Design review of the part built by this model. Coordinates are the model's own, in mm. A direction names the side the tool comes from. Round coordinates to 2 decimals unless told otherwise and drop trailing zeros. Order: outer loops, then holes, each group sorted by start corner. A loop starts at its lowest first (then second) coordinate and runs counter-clockwise, first axis right, second up. Notation, with made-up numbers: M 79,22 L 122,22 A12 ccw 122,26 Z; hole C 58,16.5 d4. An arc over 180 degrees is marked long. Use a Markdown table: item, result. Add a question column.
(1) Machinability: for faces 1 (the face through (26.877, 0.986, 63.376)), 2 (the face through (-36.96, 0.99, 55.82)), which of the approach directions +Z, -Z, +X, -X, +Y, -Y give a long, thin tool a straight path to every point of the face, cutting with its end or side? Answer none if there is none.
(2) Take a section at B-B (z = 11). Write out the cut boundary in (x, y) (3 decimals), then the cut area to 3 significant figures.
(3) Take a section at A-A (x = 47). Write out the cut boundary in (y, z), then the cut area to 3 significant figures.
(4) Take a section at D-D (y = 1.6). Count the separate pieces of the cut face and the enclosed holes in it, then the cut area to 3 significant figures.
(5) Take a section at C-C (x = -23). Write out the cut boundary in (y, z), then the cut area to 3 significant figures.
(6) To check wall thickness, follow probe 1 along Z at (x, y) = (13, 0.7); probe 2 along Z at (x, y) = (-28.5, 0.5); probe 3 along Z at (x, y) = (21.5, 0.5). State the ranges of each line that lie inside material, in increasing order. Write a range as from..to.
(7) For pin 1 (1 mm diameter, centred on y = 1, z = 217.5, fed in from +X); pin 2 (0.6 mm diameter, centred on y = 1, z = 223, fed in from -X); pin 3 (1 mm diameter, centred on y = 1, z = 165.5, fed in from +X), all flat-tipped, find the tip position at first contact; note any pin that passes through.
```python
from build123d import *

# Parameters (mm, degrees)
SKETCH1_R           = 1.5
BOSS_EXTRUDE1_DEPTH = 2
CHAMFER1_SIZE       = 2
SKETCH4_W           = 36.30312698
SKETCH4_H           = 0.486110151
CUT_EXTRUDE3_DEPTH  = 10
SKETCH5_W           = 29
SKETCH5_H           = 1.352839956
CUT_EXTRUDE4_DEPTH  = 10
SKETCH6_R           = 1.5
CUT_EXTRUDE5_DEPTH  = 2
SKETCH2_W           = 29
SKETCH2_H           = 5.227477133
CUT_EXTRUDE1_DEPTH  = 10
SKETCH7_R           = 1.5
CUT_EXTRUDE6_DEPTH  = 2
CHAMFER2_SIZE       = 2
CUT_EXTRUDE7_DEPTH  = 10
SKETCH9_W           = 2.845003066
SKETCH9_H           = 3
CUT_EXTRUDE8_DEPTH  = 2
SKETCH10_W          = 2.678834089
SKETCH10_H          = 3.000004318
BOSS_EXTRUDE2_DEPTH = 2
SKETCH11_W          = 3.5
SKETCH11_H          = 3
CUT_EXTRUDE9_DEPTH  = 2
SKETCH12_W          = 3.3
SKETCH12_H          = 23.000004318
BOSS_EXTRUDE3_DEPTH = 2
SKETCH13_W          = 2.845003066
SKETCH13_H          = 20
CUT_EXTRUDE10_DEPTH = 2
SKETCH14_R          = 1.5
CUT_EXTRUDE11_DEPTH = 2
CHAMFER3_SIZE       = 2
SKETCH15_W          = 0.991837727
SKETCH15_H          = 3
CUT_EXTRUDE12_DEPTH = 2
SKETCH16_W          = 0.826217407
SKETCH16_H          = 20.799074454
BOSS_EXTRUDE4_DEPTH = 2
SKETCH17_R          = 1.5
CUT_EXTRUDE13_DEPTH = 2
CHAMFER4_SIZE       = 2


# Some blends are built 0.0001 mm under size
with BuildPart() as part:
    # Sketch1 → Boss-Extrude1 (new body)
    with BuildSketch(Plane(origin=(0, 0, 0), x_dir=(1, 0, 0), z_dir=(0, 1, 0))):
        Polygon((0, 4.604246944), (7, 4.604246944), (7, 1.604246944), (27, 1.604246944), (27, 4.604246944), (34, 4.604246944), (34, -18.395753056), (52, -18.395753056), (52, -36.395753056), (23.933920219, -43.895753056), (29.976717731, -83.895753056), (-6.023282269, -83.895753056), (-5.667548556, -108.895753056), (23.332451444, -108.895753056), (23.332451444, -133.895753056), (18.332451444, -133.895753056), (18.332451444, -176.895753056), (16.332451444, -176.895753056), (16.332451444, -207.895753056), (24.332451444, -207.895753056), (24.332451444, -211.895753056), (31.332451444, -211.895753056), (31.332451444, -223.895753056), (24.332451444, -223.895753056), (24.332451444, -220.895753056), (4.332451444, -220.895753056), (4.332451444, -223.895753056), (-2.667548556, -223.895753056), (-2.667548556, -203.096678602), (-45.667548556, -203.096678602), (-45.667548556, -76.129309552), (-28, -34.929185263), (-28, -18.395753056), (0, -18.395753056), align=None)
        with Locations(Location((47, -23.395753056, 0), (0, 0, 270))):
            Circle(SKETCH1_R, mode=Mode.SUBTRACT)
        with Locations(Location((-23, -23.395753056, 0), (0, 0, 270))):
            Circle(SKETCH1_R, mode=Mode.SUBTRACT)
        with Locations(Location((25.976717731, -79.895753056, 0), (0, 0, 270))):
            Circle(SKETCH1_R, mode=Mode.SUBTRACT)
        with Locations(Location((6.356717731, -79.895753056, 0), (0, 0, 270))):
            Circle(SKETCH1_R, mode=Mode.SUBTRACT)
    extrude(amount=BOSS_EXTRUDE1_DEPTH)

    # Chamfer1
    # the kernel refuses this chamfer: 2 mm, written as the material it takes off along each edge
    with BuildSketch(Plane(origin=(6.356717731, 2, 79.895753056), x_dir=(0, 0, 1), z_dir=(-1, 0, 0))) as chamfer1_piece_1:
        Polygon((1.5, -CHAMFER1_SIZE), (1.5 + CHAMFER1_SIZE, 0), (1.5, 0), align=None)
    revolve(axis=Axis((6.356717731, 2, 79.895753056), (0, 1, 0)), mode=Mode.SUBTRACT)
    with BuildSketch(Plane(origin=(25.976717731, 2, 79.895753056), x_dir=(0, 0, 1), z_dir=(-1, 0, 0))) as chamfer1_piece_2:
        Polygon((1.5, -CHAMFER1_SIZE), (1.5 + CHAMFER1_SIZE, 0), (1.5, 0), align=None)
    revolve(axis=Axis((25.976717731, 2, 79.895753056), (0, 1, 0)), mode=Mode.SUBTRACT)
    with BuildSketch(Plane(origin=(-23, 2, 23.395753056), x_dir=(0, 0, 1), z_dir=(-1, 0, 0))) as chamfer1_piece_3:
        Polygon((1.5, -CHAMFER1_SIZE), (1.5 + CHAMFER1_SIZE, 0), (1.5, 0), align=None)
    revolve(axis=Axis((-23, 2, 23.395753056), (0, 1, 0)), mode=Mode.SUBTRACT)
    with BuildSketch(Plane(origin=(47, 2, 23.395753056), x_dir=(0, 0, 1), z_dir=(-1, 0, 0))) as chamfer1_piece_4:
        Polygon((1.5, -CHAMFER1_SIZE), (1.5 + CHAMFER1_SIZE, 0), (1.5, 0), align=None)
    revolve(axis=Axis((47, 2, 23.395753056), (0, 1, 0)), mode=Mode.SUBTRACT)

    # Sketch4 → Cut-Extrude3 (cut)
    with BuildSketch(Plane(origin=(0, 2, 0), x_dir=(1, 0, 0), z_dir=(0, 1, 0))):
        with Locations((12.128281221, -83.65269798)):
            Rectangle(SKETCH4_W, SKETCH4_H)
    extrude(amount=-CUT_EXTRUDE3_DEPTH, mode=Mode.SUBTRACT)

    # Sketch5 → Cut-Extrude4 (cut)
    with BuildSketch(Plane(origin=(0, 2, 0), x_dir=(1, 0, 0), z_dir=(0, 1, 0))):
        with Locations((8.832451444, -109.572173034)):
            Rectangle(SKETCH5_W, SKETCH5_H)
    extrude(amount=-CUT_EXTRUDE4_DEPTH, mode=Mode.SUBTRACT)

    # Sketch6 → Cut-Extrude5 (cut)
    with BuildSketch(Plane(origin=(0, 2, 0), x_dir=(1, 0, 0), z_dir=(0, 1, 0))):
        with Locations(Location((-28.667548556, -130.096678602, 0), (0, 0, 270))):
            Circle(SKETCH6_R)
        with Locations(Location((-28.667548556, -199.096678602, 0), (0, 0, 270))):
            Circle(SKETCH6_R)
    extrude(amount=-CUT_EXTRUDE5_DEPTH, mode=Mode.SUBTRACT)

    # Sketch2 → Cut-Extrude1 (cut)
    with BuildSketch(Plane(origin=(0, 2, 0), x_dir=(1, 0, 0), z_dir=(0, 1, 0))):
        with Locations((8.832451444, -111.509491623)):
            Rectangle(SKETCH2_W, SKETCH2_H)
    extrude(amount=-CUT_EXTRUDE1_DEPTH, mode=Mode.SUBTRACT)

    # Sketch7 → Cut-Extrude6 (cut)
    with BuildSketch(Plane(origin=(0, 2, 0), x_dir=(1, 0, 0), z_dir=(0, 1, 0))):
        with Locations(Location((20.332451444, -119.213897383, 0), (0, 0, 270))):
            Circle(SKETCH7_R)
        with Locations(Location((20.332451444, -129.213897383, 0), (0, 0, 270))):
            Circle(SKETCH7_R)
    extrude(amount=-CUT_EXTRUDE6_DEPTH, mode=Mode.SUBTRACT)

    # Chamfer2
    # the kernel refuses this chamfer: 2 mm, written as the material it takes off along each edge
    with BuildSketch(Plane(origin=(20.332451444, 0, 119.213897383), x_dir=(0, 0, 1), z_dir=(-1, 0, 0))) as chamfer2_piece_1:
        Polygon((1.5 + CHAMFER2_SIZE, 0), (1.5, CHAMFER2_SIZE), (1.5, 0), align=None)
    revolve(axis=Axis((20.332451444, 0, 119.213897383), (0, 1, 0)), mode=Mode.SUBTRACT)
    with BuildSketch(Plane(origin=(20.332451444, 0, 129.213897383), x_dir=(0, 0, 1), z_dir=(-1, 0, 0))) as chamfer2_piece_2:
        Polygon((1.5 + CHAMFER2_SIZE, 0), (1.5, CHAMFER2_SIZE), (1.5, 0), align=None)
    revolve(axis=Axis((20.332451444, 0, 129.213897383), (0, 1, 0)), mode=Mode.SUBTRACT)

    # Sketch8 → Cut-Extrude7 (cut)
    with BuildSketch(Plane(origin=(0, 2, 0), x_dir=(1, 0, 0), z_dir=(0, 1, 0))):
        Polygon((23.96091905, -43.888538253), (52, -36.395753056), (23.459204593, -40.551765872), align=None)
    extrude(amount=-CUT_EXTRUDE7_DEPTH, mode=Mode.SUBTRACT)

    # Sketch9 → Cut-Extrude8 (cut)
    with BuildSketch(Plane(origin=(0, 2, 0), x_dir=(1, 0, 0), z_dir=(0, 1, 0))):
        with Locations((32.577498467, 3.104246944)):
            Rectangle(SKETCH9_W, SKETCH9_H)
    extrude(amount=-CUT_EXTRUDE8_DEPTH, mode=Mode.SUBTRACT)

    # Sketch10 → Boss-Extrude2 (add)
    with BuildSketch(Plane(origin=(0, 2, 0), x_dir=(1, 0, 0), z_dir=(0, 1, 0))):
        with Locations((25.660582956, 3.104249103)):
            Rectangle(SKETCH10_W, SKETCH10_H)
    extrude(amount=-BOSS_EXTRUDE2_DEPTH)

    # Sketch11 → Cut-Extrude9 (cut)
    with BuildSketch(Plane(origin=(0, 2, 0), x_dir=(1, 0, 0), z_dir=(0, 1, 0))):
        with Locations((5.25, 3.104246944)):
            Rectangle(SKETCH11_W, SKETCH11_H)
    extrude(amount=-CUT_EXTRUDE9_DEPTH, mode=Mode.SUBTRACT)

    # Sketch12 → Boss-Extrude3 (add)
    with BuildSketch(Plane(origin=(0, 2, 0), x_dir=(1, 0, 0), z_dir=(0, 1, 0))):
        with Locations((-1.65, -6.895750897)):
            Rectangle(SKETCH12_W, SKETCH12_H)
    extrude(amount=-BOSS_EXTRUDE3_DEPTH)

    # Sketch13 → Cut-Extrude10 (cut)
    with BuildSketch(Plane(origin=(0, 2, 0), x_dir=(1, 0, 0), z_dir=(0, 1, 0))):
        with Locations((32.577498467, -8.395753056)):
            Rectangle(SKETCH13_W, SKETCH13_H)
    extrude(amount=-CUT_EXTRUDE10_DEPTH, mode=Mode.SUBTRACT)

    # Sketch14 → Cut-Extrude11 (cut)
    with BuildSketch(Plane.XZ):
        with Locations(Location((0.071165911, 0.895748738, 0), (0, 0, 270))):
            Circle(SKETCH14_R)
        with Locations(Location((27.571165911, 0.895748738, 0), (0, 0, 270))):
            Circle(SKETCH14_R)
    extrude(amount=-CUT_EXTRUDE11_DEPTH, mode=Mode.SUBTRACT)

    # Chamfer3
    # the kernel refuses this chamfer: 2 mm, written as the material it takes off along each edge
    with BuildSketch(Plane(origin=(0.071165911, 2, 0.895748738), x_dir=(0, 0, -1), z_dir=(-1, 0, 0))) as chamfer3_piece_1:
        Polygon((1.5 + CHAMFER3_SIZE, 0), (1.5, CHAMFER3_SIZE), (1.5, 0), align=None)
    revolve(axis=Axis((0.071165911, 2, 0.895748738), (0, -1, 0)), mode=Mode.SUBTRACT)
    with BuildSketch(Plane(origin=(27.571165911, 2, 0.895748738), x_dir=(0, 0, -1), z_dir=(-1, 0, 0))) as chamfer3_piece_2:
        Polygon((1.5 + CHAMFER3_SIZE, 0), (1.5, CHAMFER3_SIZE), (1.5, 0), align=None)
    revolve(axis=Axis((27.571165911, 2, 0.895748738), (0, -1, 0)), mode=Mode.SUBTRACT)

    # Sketch15 → Cut-Extrude12 (cut)
    with BuildSketch(Plane(origin=(0, 2, 0), x_dir=(1, 0, 0), z_dir=(0, 1, 0))):
        with Locations((3.836532581, -222.395753056)):
            Rectangle(SKETCH15_W, SKETCH15_H)
    extrude(amount=-CUT_EXTRUDE12_DEPTH, mode=Mode.SUBTRACT)

    # Sketch16 → Boss-Extrude4 (add)
    with BuildSketch(Plane(origin=(0, 2, 0), x_dir=(1, 0, 0), z_dir=(0, 1, 0))):
        with Locations((-3.08065726, -213.496215829)):
            Rectangle(SKETCH16_W, SKETCH16_H)
    extrude(amount=-BOSS_EXTRUDE4_DEPTH)

    # Sketch17 → Cut-Extrude13 (cut)
    with BuildSketch(Plane.XZ):
        with Locations(Location((27.590613723, 218.395405635, 0), (0, 0, 270))):
            Circle(SKETCH17_R)
        with Locations(Location((0.090613723, 218.395405628, 0), (0, 0, 270))):
            Circle(SKETCH17_R)
    extrude(amount=-CUT_EXTRUDE13_DEPTH, mode=Mode.SUBTRACT)

    # Chamfer4
    chamfer4_edges = [part.edges().sort_by_distance(p)[0] for p in [
        (27.590613723, 2, 219.895405635),
        (0.090613723, 2, 219.895405628),
    ]]
    chamfer(chamfer4_edges, length=CHAMFER4_SIZE - 0.0001)  # a hair under: the kernel refuses the full size


solid = part.part
```
Verdict:
| question | item | result |
|---|---|---|
| 1 | face 1 | +X, +Y, -Y |
| 1 | face 2 | -Z, -X, +Y, -Y |
| 2 | outline | M -3.3,0 L 31.155,0 L 31.155,2 L -3.3,2 Z |
| 2 | area | 68.9 mm^2 |
| 3 | outline | M 0,18.4 L 2,18.4 L 2,19.9 L 0,21.9 Z; M 0,24.9 L 2,26.9 L 2,37.12 L 0,37.12 Z |
| 3 | area | 27.5 mm^2 |
| 4 | separate pieces | 1 |
| 4 | enclosed holes | 12 |
| 4 | area | 12,500 mm^2 |
| 5 | outline | M 0,18.4 L 2,18.4 L 2,19.9 L 0,21.9 Z; M 0,24.9 L 2,26.9 L 2,203.1 L 0,203.1 Z |
| 5 | area | 359 mm^2 |
| 6 | probe 1 | z = -1.6..83.41, 114.12..220.9 |
| 6 | probe 2 | z = 36.1..128.61, 131.59..197.61, 200.59..203.1 |
| 6 | probe 3 | z = -1.6..83.41, 114.12..116.45, 121.98..126.45, 131.98..133.9, 207.9..220.9 |
| 7 | pin 1 | stops at x = 31.33 |
| 7 | pin 2 | stops at x = -3.49 |
| 7 | pin 3 | stops at x = 18.33 |
